Verification items for the finished model (mm, model axes). A direction names the side the tool comes from. Round coordinates to 2 decimals unless told otherwise and drop trailing zeros. Loops run counter-clockwise (first coordinate to the right, second up) from the corner with the lowest first, then second, coordinate; pieces in that order, holes last. Notation, with made-up numbers: M 82.25,-2 L 88.25,-2 A23 ccw 88.25,37 Z; hole C 64.25,86.25 d7. An arc over 180 degrees is marked long. One line per item, written item: value.
from build123d import *

# Parameters (mm, degrees)
BOSS_EXTRUDE1_DEPTH     = 914.4
SKETCH2_W               = 228.6
SKETCH2_H               = 304.8
CUT_EXTRUDE1_DEPTH      = 1894.961351242
CUT_EXTRUDE2_DEPTH      = 1894.961351242
CUT_EXTRUDE2_DEPTH_BACK = 1894.961351242
SKETCH3_W               = 609.6
SKETCH3_H               = 330.2


with BuildPart() as part:
    # Sketch1 → Boss-Extrude1 (new body)
    with BuildSketch(Plane.XY):
        Polygon((-381, 0), (-381, 457.2), (381, 457.2), (381, 0), (1066.8, 0), (1066.8, 304.8), (508, 1270), (-508, 1270), (-1066.8, 304.8), (-1066.8, 0), align=None)
    extrude(amount=-BOSS_EXTRUDE1_DEPTH)

    # Sketch2 → Cut-Extrude1 (cut, through all)
    with BuildSketch(Plane(origin=(0, 0, 0), x_dir=(1, 0, 0), z_dir=(0, 1, 0))):
        with Locations((-952.5, 152.4)):
            Rectangle(SKETCH2_W, SKETCH2_H)
        with Locations((952.5, 152.4)):
            Rectangle(SKETCH2_W, SKETCH2_H)
    extrude(amount=CUT_EXTRUDE1_DEPTH, mode=Mode.SUBTRACT)

    # Sketch3 → Cut-Extrude2 (cut, two sides: drawn at the far end of the back side and taken through both)
    with BuildSketch(Plane(origin=(0, 0, 0), x_dir=(0, 0, -1), z_dir=(1, 0, 0)).offset(-CUT_EXTRUDE2_DEPTH_BACK)):
        with Locations((304.8, 1104.9)):
            Rectangle(SKETCH3_W, SKETCH3_H)
    extrude(amount=CUT_EXTRUDE2_DEPTH + CUT_EXTRUDE2_DEPTH_BACK, mode=Mode.SUBTRACT)


solid = part.part
(1) Thickness scan on L1, parallel to X at y = 400.5, z = -101.5; L2, parallel to X at y = 54.5, z = -851; L3, parallel to Y at x = 30.5, z = -88. Record the ranges inside material, lowest first. Write a range as from..to.
Completed:
L1: x = -838.2..-381, 381..838.2
L2: x = -1066.8..-381, 381..1066.8
L3: y = 457.2..939.8
(2) Sectioned sample at C-C on y = 552.5. Enter the section's corners in (x, z), and give its area (3 significant figures).
Completed:
outline: M -923.39,-914.4 L 923.39,-914.4 L 923.39,-304.8 L 838.2,-304.8 L 838.2,0 L -838.2,0 L -838.2,-304.8 L -923.39,-304.8 Z
area: 1,640,000 mm^2
(3) Sectioned sample at B-B on z = -180.5. Enter the section's corners in (x, y), and give its area (3 significant figures).
Completed:
outline: M -838.2,0 L -381,0 L -381,457.2 L 381,457.2 L 381,0 L 838.2,0 L 838.2,699.65 L 699.17,939.8 L -699.17,939.8 L -838.2,699.65 Z
area: 1,190,000 mm^2
(4) Sectioned sample at A-A on x = 410.5. Enter the section's corners in (y, z).
Completed:
outline: M 0,-914.4 L 1270,-914.4 L 1270,-609.6 L 939.8,-609.6 L 939.8,0 L 0,0 Z
(5) Tool access check on faces 5 (the face through (838.2, 345, -150)), 6 (the face through (-10, 939.8, -301)), 7 (the face through (-381, 225, -451)), 8 (the face through (-838.2, 345, -150)), 9 (the face through (-15, 644, -914.4)). Record the directions out of +Z, -Z, +X, -X, +Y, -Y that give a thin tool (end or side, any length) a straight path to the whole face; none if there is none.
Completed:
face 5: +Z, +X, +Y, -Y
face 6: +Z, +X, -X, +Y
face 7: +Z, -Z, -Y
face 8: +Z, -X, +Y, -Y
face 9: -Z, +X, -X, +Y, -Y
(6) Depth check by flat-ended pin: pin 1 Ø2 at (y, z) = (332, -722.5) entering from -X; pin 2 Ø6 at (x, z) = (187.5, -497) entering from -Y; pin 3 Ø10 at (y, z) = (508.5, -124.5) entering from +X; pin 4 Ø2 at (x, y) = (183, 926) entering from +Z. Enter the tip coordinate at first touch or a pass-through.
Completed:
pin 1: stops at x = -1051.63
pin 2: stops at y = 457.2
pin 3: stops at x = 838.2
pin 4: stops at z = 0
(7) Sectioned sample at D-D on y = 383. Enter the section's corners in (x, z), and give its area (3 significant figures).
Completed:
outline: M -1021.53,-914.4 L -381,-914.4 L -381,0 L -838.2,0 L -838.2,-304.8 L -1021.53,-304.8 Z; M 381,-914.4 L 1021.53,-914.4 L 1021.53,-304.8 L 838.2,-304.8 L 838.2,0 L 381,0 Z
area: 1,060,000 mm^2
(8) Mould release check, pull along X, two halves, no side actions. Record for faces 1 (the face through (381, 232, -451)), 2 (the face through (1066.8, 150, -605)), 3 (the face through (-5, 457.2, -451)), 4 (the face through (-929, 267, -304.8)): +X half, -X half, draft (parallel to the pull), parting line (faces both ways), or undercut.
Completed:
face 1: undercut
face 2: +X half
face 3: undercut
face 4: draft
